from build123d import *

# Parameters (mm, degrees)
SKETCH1_W               = 19.05
SKETCH1_H               = 15.08125
BOARD_DEPTH             = 2
SKETCH2_R               = 2.778125
LASERBARREL_DEPTH       = 10
SKETCH4_W               = 2.25
SKETCH4_H               = 5.55
BARREL_BUTT_MOUNT_DEPTH = 3.175
BOSS_EXTRUDE1_DEPTH     = 0.325
LPATTERN1_COUNT         = 2
LPATTERN1_PITCH         = 2.54
LPATTERN1_COL_COUNT     = 2
LPATTERN1_COL_PITCH     = 2.54
SKETCH6_R               = 1.625
CUT_EXTRUDE1_DEPTH      = 1


with BuildPart() as part:
    # Sketch1 → Board (new body)
    with BuildSketch(Plane(origin=(0, 0, 0), x_dir=(1, 0, 0), z_dir=(0, 1, 0))):
        Rectangle(SKETCH1_W, SKETCH1_H)
    extrude(amount=BOARD_DEPTH)



with BuildPart() as body_2:
    # Sketch2 → LaserBarrel (new body)
    with BuildSketch(Plane(origin=(12.7, 0, 0), x_dir=(0, 0, -1), z_dir=(1, 0, 0))):
        with Locations((1.190625, 4.85)):
            Circle(SKETCH2_R)
    extrude(amount=-LASERBARREL_DEPTH)


with BuildPart() as part_1:
    add(part.part)

    add(body_2.part)  # Barrel Butt Mount merges body 2
    # Sketch4 → Barrel Butt Mount (add)
    with BuildSketch(Plane.ZY.offset(-2.7)):
        with Locations((-1.190625, 4.775)):
            Rectangle(SKETCH4_W, SKETCH4_H)
    extrude(amount=BARREL_BUTT_MOUNT_DEPTH)

    # Sketch5 → Boss-Extrude1 (add, symmetric)
    with BuildSketch(Plane.XY):
        Polygon((-7.025, 2), (-6.375, 2), (-6.375, 4.844974747), (-7.180025253, 5.65), (-13.180025253, 5.65), (-13.180025253, 5), (-7.449264069, 5), (-7.025, 4.575735931), align=None)
    boss_extrude1 = extrude(amount=BOSS_EXTRUDE1_DEPTH, both=True)

    # LPattern1: Boss-Extrude1 ×2
    with Locations(*[(0, 0, -i * LPATTERN1_PITCH) for i in range(1, LPATTERN1_COUNT)]):
        add(boss_extrude1)

    # LPattern1 col: Boss-Extrude1 ×2
    with Locations(*[(0, 0, i * LPATTERN1_COL_PITCH) for i in range(1, LPATTERN1_COL_COUNT)]):
        add(boss_extrude1)

    # Sketch6 → Cut-Extrude1 (cut)
    with BuildSketch(Plane(origin=(12.7, 0, 0), x_dir=(0, 0, -1), z_dir=(1, 0, 0))):
        with Locations((1.190625, 4.85)):
            Circle(SKETCH6_R)
    extrude(amount=-CUT_EXTRUDE1_DEPTH, mode=Mode.SUBTRACT)


solid = part_1.part
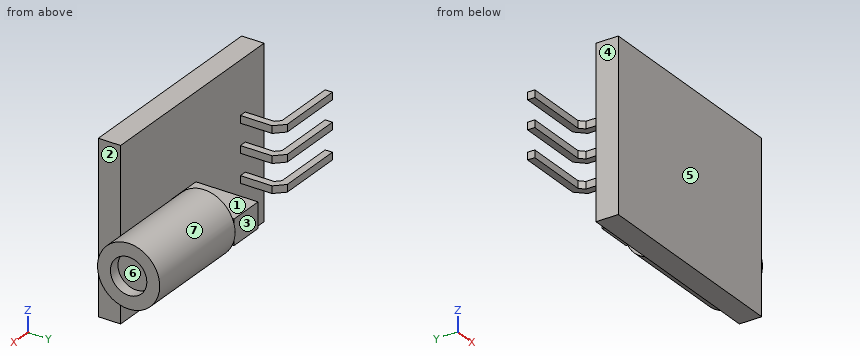
Geometry: final body of the model. Coordinates: model frame, mm. Face numbers are marked on the shaded views. A direction names the side the tool comes from. Coordinates: 2 decimals unless noted, no trailing zeros. Loops run counter-clockwise (first coordinate to the right, second up) from the corner with the lowest first, then second, coordinate; pieces in that order, holes last. Notation, with made-up numbers: (43.25, 26) - (49.25, 26) arc R20 ccw to (49.25, 42) - close; hole circle Ø7 at (21, -14.5). An arc over 180 degrees is marked (long way). Put each result on its own line as item: value. Start each with the question number.
Q1. Cut plane B-B, the plane x = 5. Return loops of the section in (y, z), and give its area (3 significant figures).
Q2. Pin query (flat end, axial travel): pin 1 Ø0.7 at (x, z) = (-9.5, -2.5) entering from +Y; pin 2 Ø1.1 at (x, y) = (-8.5, 3.5) entering from +Z; pin 3 Ø3 at (x, y) = (2.5, 5) entering from -Z; pin 4 Ø0.5 at (y, z) = (3, 2.5) entering from +X (3 decimals). Return the tip coordinate at first contact, or that it passes through.
Q3. Pull-direction query (Y, two-part tool) for the marked faces 4, 5, 6 and 7; classes: released by +Y, released by -Y, zero draft, split by the parting line, or undercut.
Q4. Cut plane A-A, the plane x = -11. Return loops of the section in (y, z) (3 decimals).
Q5. Set-up query: the marked faces 1, 2 and 3. Return all of +Z, -Z, +X, -X, +Y, -Y with unobstructed straight access to the full face (end or side cutting, diameter ignored); none if empty.
Q6. Cut plane C-C, the plane z = -3.25. Return loops of the section in (x, y) (3 decimals).
Q7. Line query: line 1 (Z direction, x = -12, y = 5.5) (3 decimals); line 2 (X direction, y = 2.75, z = 0.5); line 3 (X direction, y = 6, z = -1.25) (3 decimals). Output: solid intervals per line, ascending.
Q8. Cut plane D-D, the plane z = 6. Return loops of the section in (x, y) (3 decimals), and give its area (3 significant figures).
Filled sheet:
1. outline: (0, -7.54) - (2, -7.54) - (2, 7.54) - (0, 7.54) - close; circle Ø5.56 at (4.85, -1.19)
1. area: 54.4 mm²
2. pin 1: y = 5.65
2. pin 2: through
2. pin 3: z = -3.97
2. pin 4: x = -6.375
3. face 4: zero draft
3. face 5: released by -Y
3. face 6: undercut
3. face 7: undercut
4. outline: (5, -2.865) - (5.65, -2.865) - (5.65, -2.215) - (5, -2.215) - close; (5, -0.325) - (5.65, -0.325) - (5.65, 0.325) - (5, 0.325) - close; (5, 2.215) - (5.65, 2.215) - (5.65, 2.865) - (5, 2.865) - close
5. face 1: +Z, +Y
5. face 2: +Z, -Z, +X, -Y
5. face 3: +Z, -Z, -X, +Y
6. outline: (-9.525, 0) - (9.525, 0) - (9.525, 2) - (-9.525, 2) - close; (2.7, 2.985) - (12.7, 2.985) - (12.7, 6.715) - (2.7, 6.715) - close
7. line 1: -2.865 to -2.215, -0.325 to 0.325, 2.215 to 2.865
7. line 2: 2.7 to 12.7
7. line 3: -0.475 to 11.7
8. outline: (-9.525, 0) - (9.525, 0) - (9.525, 2) - (-9.525, 2) - close
8. area: 38.1 mm²
